Check sheet for the modelled part. Datum: model origin and axes. Units: mm. A direction names the side the tool comes from. Coordinates: 2 decimals unless noted, no trailing zeros. Order: outer loops, then holes, each group sorted by start corner. A loop starts at its lowest first (then second) coordinate and runs counter-clockwise, first axis right, second up. Notation, with made-up numbers: M 85.25,-16 L 107.25,-16 A32 cw 107.25,20 Z; hole C 14,0 d6. An arc over 180 degrees is marked long. Answer in a Markdown table with one row per item. Add a question column.
from build123d import *

# Parameters (mm, degrees)
SKETCH1_W           = 416.3
SKETCH1_H           = 387.782
BOSS_EXTRUDE1_DEPTH = 7.5
SKETCH3_W           = 50
SKETCH3_H           = 80
BOSS_EXTRUDE2_DEPTH = 76.2
SKETCH5_R           = 15.5
CUT_EXTRUDE1_DEPTH  = 410.077660574
SKETCH6_R           = 15.5
CUT_EXTRUDE2_DEPTH  = 315.576433289


with BuildPart() as part:
    # Sketch1 → Boss-Extrude1 (new, symmetric)
    with BuildSketch(Plane.XY):
        Rectangle(SKETCH1_W, SKETCH1_H)
    extrude(amount=BOSS_EXTRUDE1_DEPTH, both=True)

    # Sketch3 → Boss-Extrude2 (add)
    with BuildSketch(Plane(origin=(0, 0, -7.5), x_dir=(-1, 0, 0), z_dir=(0, 0, -1))):
        with Locations((117.2, 100)):
            Rectangle(SKETCH3_W, SKETCH3_H)
        with Locations((117.2, -100)):
            Rectangle(SKETCH3_W, SKETCH3_H)
        with Locations((-117.2, -100)):
            Rectangle(SKETCH3_W, SKETCH3_H)
        with Locations((-117.2, 100)):
            Rectangle(SKETCH3_W, SKETCH3_H)
        Rectangle(SKETCH3_W, SKETCH3_H)
    extrude(amount=BOSS_EXTRUDE2_DEPTH)

    # Sketch5 → Cut-Extrude1 (cut, through all)
    with BuildSketch(Plane.ZY.offset(142.2)):
        with Locations(Location((-45.6, 100, 0), (0, 0, 270))):
            Circle(SKETCH5_R)
        with Locations(Location((-45.6, -100, 0), (0, 0, 270))):
            Circle(SKETCH5_R)
    extrude(amount=-CUT_EXTRUDE1_DEPTH, mode=Mode.SUBTRACT)

    # Sketch6 → Cut-Extrude2 (cut, through all)
    with BuildSketch(Plane(origin=(25, 0, 0), x_dir=(0, 0, -1), z_dir=(1, 0, 0))):
        with Locations(Location((45.6, 0, 0), (0, 0, 90))):
            Circle(SKETCH6_R)
    extrude(amount=-CUT_EXTRUDE2_DEPTH, mode=Mode.SUBTRACT)


solid = part.part
1. Set-up check for faces 5 (the flat face through (92.2, -101, -62)), 6 (the flat face through (142.2, 99, -62)), 7 (the flat face through (0, 40, -45)), 8 (the flat face through (-25, -1, -62)): record each of +Z, -Z, +X, -X, +Y, -Y from which the full face is reachable in a straight line by a thin tool's end or side.
2. Section check B-B on x = 111. Enter the section's corners in (y, z), then the cut area to 3 significant figures.
3. Release check for a two-part mould opening along Z. For faces 1 (the flat face through (118, 101, -83.7)), 2 (the cylindrical face through (-117.55, -87.7, -55.03)), 3 (the flat face through (-117, -140, -45)), 4 (the flat face through (-3, 3, 7.5)) record: released by +Z, released by -Z, zero draft, split by the parting line, or undercut.
4. Scan lines: line 1 (Y direction, x = -126, z = -45); line 2 (Y direction, x = -97.5, z = -14.5); line 3 (X direction, y = 112.5, z = -23). Record each from-to range of solid material in increasing order.
5. Section check A-A on z = -72. Enter the section's corners in (x, y).
6. Go/stop test with flat-tipped pins: pin 1 Ø3 at (y, z) = (-66, -40.5) entering from +X; pin 2 Ø3 at (y, z) = (-68, -31.5) entering from -X; pin 3 Ø5 at (x, y) = (-22, 84) entering from -Z. Record where each tip stops, or that it passes through.
7. Section check C-C on y = 100. Enter the section's corners in (x, z), then the cut area to 3 significant figures.
8. Section check D-D on x = -7. Enter the section's corners in (y, z).
Result sheet:
| question | item | result |
|---|---|---|
| 1 | face 5 | -Z, +Y, -Y |
| 1 | face 6 | -Z, +X, +Y, -Y |
| 1 | face 7 | -Z, +X, -X, +Y |
| 1 | face 8 | -Z, -X, +Y, -Y |
| 2 | outline | M -193.89,-7.5 L -140,-7.5 L -140,-83.7 L -60,-83.7 L -60,-7.5 L 60,-7.5 L 60,-83.7 L 140,-83.7 L 140,-7.5 L 193.89,-7.5 L 193.89,7.5 L -193.89,7.5 Z; hole C -100,-45.6 d31; hole C 100,-45.6 d31 |
| 2 | area | 16,500 mm^2 |
| 3 | face 1 | released by -Z |
| 3 | face 2 | undercut |
| 3 | face 3 | zero draft |
| 3 | face 4 | released by +Z |
| 4 | line 1 | -140 to -115.49, -84.51 to -60, 60 to 84.51, 115.49 to 140 |
| 4 | line 2 | -140 to -60, 60 to 140 |
| 4 | line 3 | -142.2 to -92.2, 92.2 to 142.2 |
| 5 | outline | M -142.2,-140 L -92.2,-140 L -92.2,-60 L -142.2,-60 Z; M -142.2,60 L -92.2,60 L -92.2,140 L -142.2,140 Z; M -25,-40 L 25,-40 L 25,40 L -25,40 Z; M 92.2,-140 L 142.2,-140 L 142.2,-60 L 92.2,-60 Z; M 92.2,60 L 142.2,60 L 142.2,140 L 92.2,140 Z |
| 6 | pin 1 | x = 142.2 |
| 6 | pin 2 | x = -142.2 |
| 6 | pin 3 | z = -7.5 |
| 7 | outline | M -208.15,-7.5 L -142.2,-7.5 L -142.2,-30.1 L -92.2,-30.1 L -92.2,-7.5 L 92.2,-7.5 L 92.2,-30.1 L 142.2,-30.1 L 142.2,-7.5 L 208.15,-7.5 L 208.15,7.5 L -208.15,7.5 Z; M -142.2,-83.7 L -92.2,-83.7 L -92.2,-61.1 L -142.2,-61.1 Z; M 92.2,-83.7 L 142.2,-83.7 L 142.2,-61.1 L 92.2,-61.1 Z |
| 7 | area | 10,800 mm^2 |
| 8 | outline | M -193.89,-7.5 L -40,-7.5 L -40,-83.7 L 40,-83.7 L 40,-7.5 L 193.89,-7.5 L 193.89,7.5 L -193.89,7.5 Z; hole C 0,-45.6 d31 |
